Can you work these out from the model? Positions are in its coordinate system, mm. A direction names the side the tool comes from. Coordinates: 2 decimals unless noted, no trailing zeros. Loops run counter-clockwise (first coordinate to the right, second up) from the corner with the lowest first, then second, coordinate; pieces in that order, holes last. Notation, with made-up numbers: M 82.25,-32 L 98.25,-32 A17 cw 98.25,-1 Z; hole C -9.75,77 d2. An arc over 180 degrees is marked long. Answer as a JSON object with one key per item and string values. Group by question number.
Item 1: Suppose I cut it at B-B (y = -501). Write out the boundary of the cut face in (x, z) (3 decimals).
Item 2: Suppose I cut it at C-C (x = 9.5). Write out the boundary of the cut face in (y, z) (3 decimals), then the cut area to 3 significant figures.
Item 3: Suppose I cut it at A-A (z = 18). Write out the boundary of the cut face in (x, y) (3 decimals), then the cut area to 3 significant figures.
Item 4: I'm going to push flat-ended pins straight in: pin 1 Ø4 at (x, z) = (27, 3) entering from +Y; pin 2 Ø2 at (x, y) = (29, -256) entering from +Z. Where does each tip first touch, or does it pass through?
Item 5: We'd pull the mould along X, two halves only. Please class faces 1 (the flat face through (22, -301, 0)), 2 (the flat face through (22, 0, -1)), 3 (the flat face through (44.45, -309, 10)): +X half, -X half, draft (parallel to the pull), parting line (faces both ways), or undercut.
Item 6: If I drill on line 1 (X direction, y = -596.9, z = -2.3); line 2 (X direction, y = -409, z = 17.25) (3 decimals); line 3 (Z direction, x = 23.5, y = -468) (3 decimals), over which ranges is the centre line in solid material (lowest first)?
Item 7: Which directions (+Z, -Z, +X, -X, +Y, -Y) give clear straight access to the entire face, cutting with the end or side of a thin tool? Please do faces 4 (the flat face through (22, -301, -3.175)), 5 (the flat face through (41.275, -309, 11)).
```python
from build123d import *

# Parameters (mm, degrees)
F0_W     = 3.175
F0_H     = 609.6
F0_W_2   = 38.1
F0_R     = 3.175
F1_DEPTH = 3.175
F2_DEPTH = 22.225


with BuildPart() as f1:
    # F0 (on Top) → F1 (new body)
    with BuildSketch(Plane.XY):
        with Locations((1.5875, -304.8)):
            Rectangle(F0_W, F0_H)
        with Locations((22.225, -304.8)):
            Rectangle(F0_W_2, F0_H)
        with Locations((22.225, -596.9)):
            Circle(F0_R, mode=Mode.SUBTRACT)
        with Locations((22.225, -12.7)):
            Circle(F0_R, mode=Mode.SUBTRACT)
        with Locations((42.8625, -304.8)):
            Rectangle(F0_W, F0_H)
    extrude(amount=-F1_DEPTH)

    # F0 (on Top) → F2 (join)
    with BuildSketch(Plane.XY):
        with Locations((1.5875, -304.8)):
            Rectangle(F0_W, F0_H)
        with Locations((42.8625, -304.8)):
            Rectangle(F0_W, F0_H)
    extrude(amount=F2_DEPTH)


solid = f1.part
```
From the geometry:
{
 "1": {"outline": "M 0,-3.175 L 44.45,-3.175 L 44.45,22.225 L 41.275,22.225 L 41.275,0 L 3.175,0 L 3.175,22.225 L 0,22.225 Z"},
 "2": {"outline": "M -609.6,-3.175 L 0,-3.175 L 0,0 L -609.6,0 Z", "area": "1,940 mm2"},
 "3": {"outline": "M 0,-609.6 L 3.175,-609.6 L 3.175,0 L 0,0 Z; M 41.275,-609.6 L 44.45,-609.6 L 44.45,0 L 41.275,0 Z", "area": "3,870 mm2"},
 "4": {"pin 1": "through", "pin 2": "z = 0"},
 "5": {"face 1": "undercut", "face 2": "draft", "face 3": "+X half"},
 "6": {"line 1": "0 to 19.05, 25.4 to 44.45", "line 2": "0 to 3.175, 41.275 to 44.45", "line 3": "-3.175 to 0"},
 "7": {"face 4": "-Z, +X, -X, +Y, -Y", "face 5": "+Z, +Y, -Y"}
}
